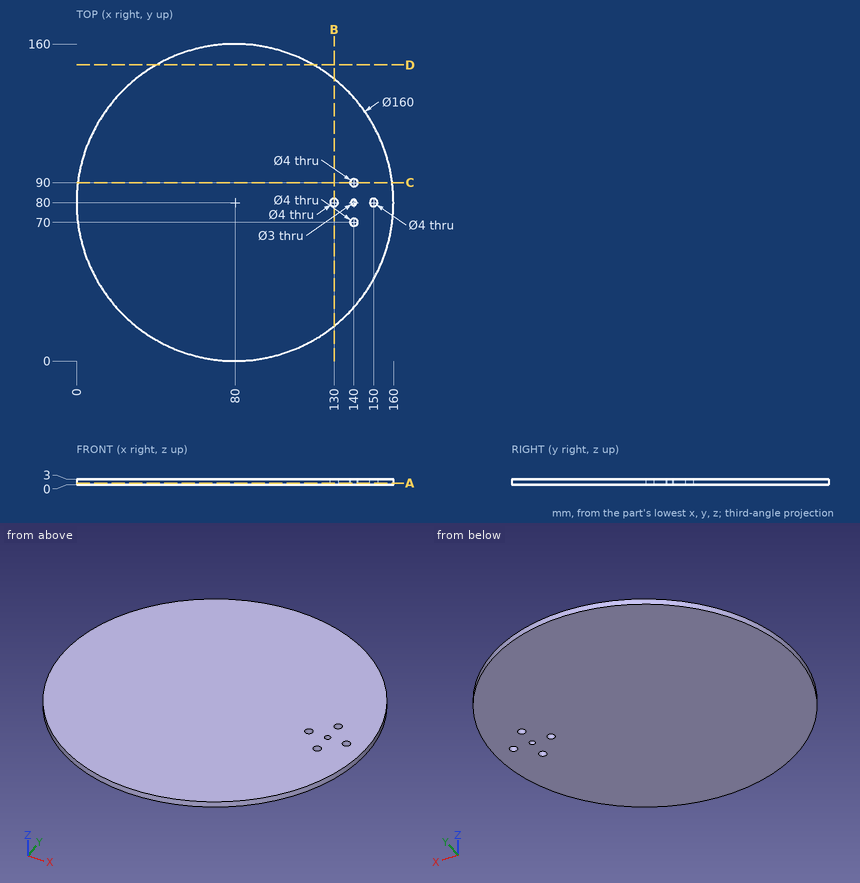
For this review, use the dimensioned drawing (mm, ordinates from the lowest corner) and the shaded views. Round coordinates to 2 decimals unless told otherwise and drop trailing zeros. Order: outer loops, then holes, each group sorted by start corner. A loop starts at its lowest first (then second) coordinate and runs counter-clockwise, first axis right, second up. Notation, with made-up numbers: (8, 53.5) - (27, 53.5) arc R23 ccw to (27, 63.5) - close; hole circle Ø3 at (57, 31.25). An arc over 180 degrees is marked (long way). Use one line per item in the form item = value.
Q1. Add section D-D on y = 149.5. Give the boundary of the cut face in (x, z), then the cut area to 3 significant figures.
Response values:
outline = (40.38, 0) - (119.62, 0) - (119.62, 3) - (40.38, 3) - close
area = 238 mm^2
Q2. Add section A-A on z = 0.95. Give the boundary of the cut face in (x, y).
Response values:
outline = circle Ø160 at (80, 80); hole circle Ø4 at (130, 80); hole circle Ø4 at (140, 70); hole circle Ø4 at (140, 90); hole circle Ø3 at (140, 80); hole circle Ø4 at (150, 80)
Q3. Add section B-B on x = 130. Give the boundary of the cut face in (y, z), then the cut area to 3 significant figures.
Response values:
outline = (17.55, 0) - (78, 0) - (78, 3) - (17.55, 3) - close; (82, 0) - (142.45, 0) - (142.45, 3) - (82, 3) - close
area = 363 mm^2
Q4. Clearance check with a flat-ended pin moving along its axis: P1, Ø1, axis at x = 80.5, z = 0.5, coming from the +Y side. State where the tip first meets the part, or that it passes through.
Response values:
P1 = 160
Q5. Add section C-C on y = 90. Give the boundary of the cut face in (x, z), then the cut area to 3 significant figures.
Response values:
outline = (0.63, 0) - (138, 0) - (138, 3) - (0.63, 3) - close; (142, 0) - (159.37, 0) - (159.37, 3) - (142, 3) - close
area = 464 mm^2
Q6. To check wall thickness, follow line 1 (Y direction, x = 140, z = 0.7); line 2 (Y direction, x = 81, z = 1.55); line 3 (X direction, y = 69, z = 0.6). State the ranges of each line that lie inside material, in increasing order.
Response values:
line_1 = 27.08 to 68, 72 to 78.5, 81.5 to 88, 92 to 132.92
line_2 = 0.01 to 159.99
line_3 = 0.76 to 138.27, 141.73 to 159.24
